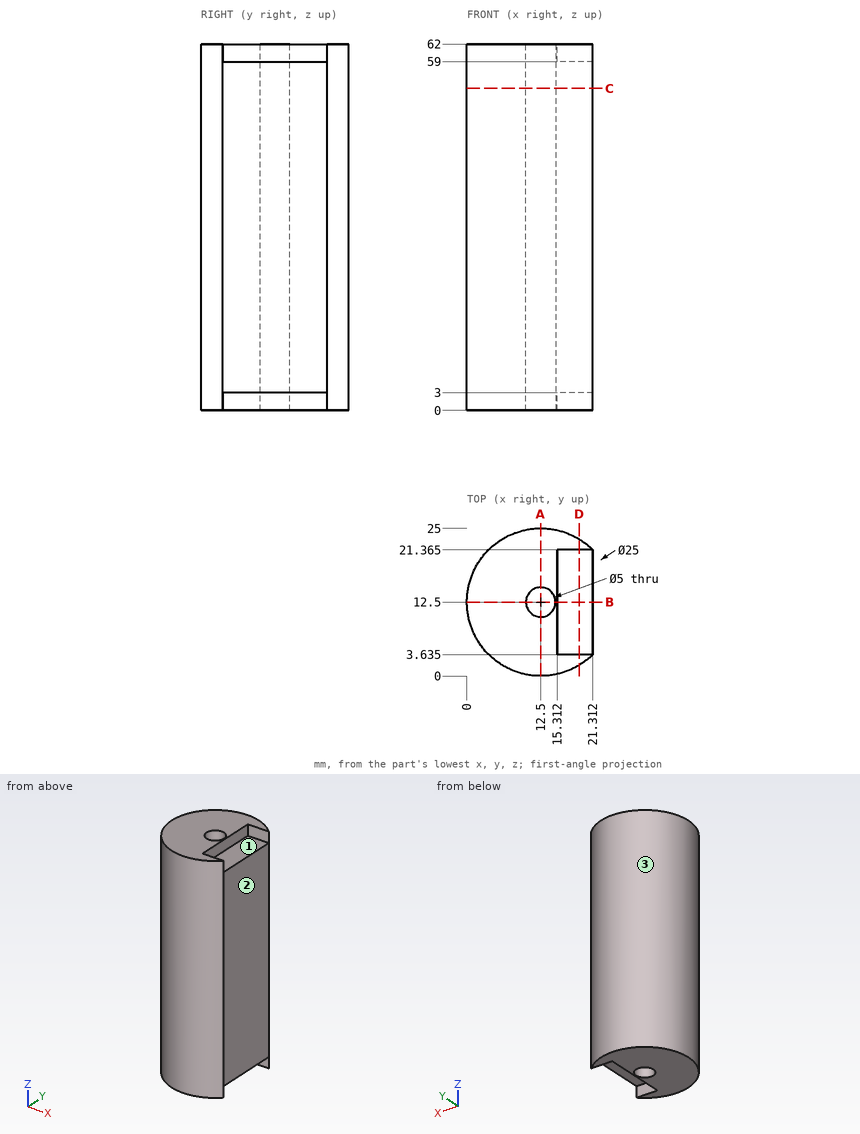
Design review of the part shown in the three views and the two pictorial views. Dimensions are in mm from the part's minimum x, y and z. Coordinates: 2 decimals unless noted, no trailing zeros. Loops run counter-clockwise (first coordinate to the right, second up) from the corner with the lowest first, then second, coordinate; pieces in that order, holes last. Notation, with made-up numbers: (34, 42) - (92, 42) arc R10 cw to (92, 48) - close; hole circle Ø4 at (-37.75, 36.5). An arc over 180 degrees is marked (long way). Use a Markdown table: item, result. Add a question column.
Item 1: We need section D-D (x = 19). Give the boundary of the cut face in (y, z) (1 decimal), and give its area (3 significant figures).
Item 2: We need section B-B (y = 12.5). Give the boundary of the cut face in (x, z).
Item 3: Insertion check: pin 1 Ø1.5 at (x, z) = (19.5, 1.5) entering from -Y (1 decimal); pin 2 Ø1.8 at (x, y) = (19, 16) entering from -Z; pin 3 Ø1.5 at (x, z) = (17, 60.5) entering from +Y. Each pin has a flat end and moves straight along its axis. Give the tip position at first contact, or say it passes through.
Item 4: Mouldability with a two-part tool opening along Y and no side actions: class the marked faces 1, 2 and 3 as pulls with the +Y half, pulls with the -Y half, needs draft (parallel to the pull), parting line crosses it, or undercut.
Item 5: We need section A-A (x = 12.5). Give the boundary of the cut face in (y, z).
Item 6: We need section C-C (z = 54.5). Give the boundary of the cut face in (x, y) (1 decimal).
Item 7: For line 1 (Y direction, x = 12.5, z = 13); line 2 (Y direction, x = 16, z = 59.5) (1 decimal); line 3 (Z direction, x = 18.5, y = 13.75), list the stretches that pass through material, from the lowest coordinate up.
Results list:
| question | item | result |
|---|---|---|
| 1 | outline | (1.8, 0) - (3.6, 0) - (3.6, 3) - (21.4, 3) - (21.4, 0) - (23.2, 0) - (23.2, 62) - (21.4, 62) - (21.4, 59) - (3.6, 59) - (3.6, 62) - (1.8, 62) - close |
| 1 | area | 1,220 mm^2 |
| 2 | outline | (0, 0) - (10, 0) - (10, 62) - (0, 62) - close; (15, 0) - (15.31, 0) - (15.31, 3) - (21.31, 3) - (21.31, 59) - (15.31, 59) - (15.31, 62) - (15, 62) - close |
| 3 | pin 1 | stops at y = 1.7 |
| 3 | pin 2 | stops at z = 3 |
| 3 | pin 3 | stops at y = 24.42 |
| 4 | face 1 | undercut |
| 4 | face 2 | needs draft |
| 4 | face 3 | parting line crosses it |
| 5 | outline | (0, 0) - (10, 0) - (10, 62) - (0, 62) - close; (15, 0) - (25, 0) - (25, 62) - (15, 62) - close |
| 6 | outline | (21.3, 3.6) - (21.3, 21.4) arc R12.5 ccw (long way) to start; hole circle Ø5 at (12.5, 12.5) |
| 7 | line 1 | y = 0 to 10, 15 to 25 |
| 7 | line 2 | y = 0.5 to 3.6, 21.4 to 24.5 |
| 7 | line 3 | z = 3 to 59 |
